The listing builds one solid part. Answer for the finished solid, in the listing's coordinates (mm). A direction names the side the tool comes from. Coordinates: 2 decimals unless noted, no trailing zeros. Order: outer loops, then holes, each group sorted by start corner. A loop starts at its lowest first (then second) coordinate and runs counter-clockwise, first axis right, second up. Notation, with made-up numbers: (-16.75, 83.5) -> (32.25, 83.5) arc R35 cw to (32.25, 121.5) -> close; hole circle Ø11 at (44.5, 60). An arc over 180 degrees is marked (long way). Write item = value, one per line.
from build123d import *

# Parameters (mm, degrees)
BOSS_EXTRUDE1_DEPTH = 17
FILLET1_R           = 1
SHELL1_T            = -3


with BuildPart() as part:
    # Sketch1 → Boss-Extrude1 (new body)
    with BuildSketch(Plane.XY):
        Polygon((0, 0), (30, 0), (30, -5), (25, -5), (5, -25), (5, -30), (0, -30), align=None)
    extrude(amount=-BOSS_EXTRUDE1_DEPTH)

    # Fillet1
    fillet1_edges = [part.edges().sort_by_distance(p)[0] for p in [
        (0, 0, -8.5),
        (30, 0, -8.5),
        (0, -30, -8.5),
        (15, 0, -17),
        (0, -15, -17),
        (15, 0, 0),
        (0, -15, 0),
    ]]
    fillet(fillet1_edges, radius=FILLET1_R)

    # Shell1
    shell1_openings = [part.faces().sort_by_distance(p)[0] for p in [
        (27.5, -5, -8.5),
        (15, -15, -8.5),
        (5, -27.5, -8.5),
    ]]
    offset(amount=SHELL1_T, openings=shell1_openings)


solid = part.part
Q1. Section D-D, the plane z = -4.75 is taken. Give the vertices of the cut face in (x, y).
The answers:
outline = (0, -29) arc R1 ccw to (1, -30) -> (5, -30) -> (5, -27) -> (3, -27) -> (3, -3) -> (27, -3) -> (27, -5) -> (30, -5) -> (30, -1) arc R1 ccw to (29, 0) -> (1, 0) arc R1 ccw to (0, -1) -> close
Q2. A tool of negligible diameter and unlimited length cuts with its end or side. For faces 5 (the face through (5, -28, -8)), 6 (the face through (0.285, -15.297, -16.699)), 7 (the face through (10, -9, -3)), 8 (the face through (4, -27, -8)), from which of +Z, -Z, +X, -X, +Y, -Y can it reach the whole face along a straight path? Write none if from no direction.
The answers:
face_5 = +Z, -Z, +X, -Y
face_6 = -Z, -X, +Y, -Y
face_7 = none
face_8 = +X
Q3. Section A-A, the plane y = -4 is taken. Give the vertices of the cut face in (x, z).
The answers:
outline = (0, -16) arc R1 ccw to (1, -17) -> (30, -17) -> (30, 0) -> (1, 0) arc R1 ccw to (0, -1) -> close; hole (3, -14) -> (27, -14) -> (27, -3) -> (3, -3) -> close
Q4. Section C-C, the plane y = -26 is taken. Give the vertices of the cut face in (x, z).
The answers:
outline = (0, -16) arc R1 ccw to (1, -17) -> (5, -17) -> (5, -14) -> (3, -14) -> (3, -3) -> (5, -3) -> (5, 0) -> (1, 0) arc R1 ccw to (0, -1) -> close
Q5. The mould has two halves that part along Y. Classify faces 1 (the face through (3, -30, -8)), 2 (the face through (3, -15, -8)), 3 (the face through (15.703, -0.285, -0.301)), 4 (the face through (0.285, -15.297, -0.301)): released by +Y, released by -Y, zero draft, split by the parting line, or undercut.
The answers:
face_1 = released by -Y
face_2 = undercut
face_3 = released by +Y
face_4 = zero draft
Q6. Each of these flat-tipped pins is pushed along its axis until it touches: pin 1 Ø3 at (x, z) = (25, -10.5) entering from -Y; pin 2 Ø5.5 at (y, z) = (-17.5, -7) entering from +X; pin 3 Ø1.5 at (y, z) = (-26.5, -8.5) entering from +X. Where does it stop, or does it pass through?
The answers:
pin_1 = -3
pin_2 = 3
pin_3 = 5
Q7. Section B-B, the plane x = 20.25 is taken. Give the vertices of the cut face in (y, z), plus the area to 3 significant figures.
The answers:
outline = (-9.75, -17) -> (-1, -17) arc R1 ccw to (0, -16) -> (0, -1) arc R1 ccw to (-1, 0) -> (-9.75, 0) -> (-9.75, -3) -> (-3, -3) -> (-3, -14) -> (-9.75, -14) -> close
area = 91.1 mm2
Q8. Find the intervals of material crossed by line 1 along Z through (x, y) = (16.75, -4.25); line 2 along X through (y, z) = (-4, -12.5); line 3 along Y through (x, z) = (4.5, -11.75), in increasing order.
The answers:
line_1 = -17 to -14, -3 to 0
line_2 = 0 to 3, 27 to 30
line_3 = -30 to -27, -3 to 0
